Geometry check sheet. Reference: the model listing, model coordinates, mm. A direction names the side the tool comes from. Coordinates: 2 decimals unless noted, no trailing zeros. Loops run counter-clockwise (first coordinate to the right, second up) from the corner with the lowest first, then second, coordinate; pieces in that order, holes last.
from build123d import *

# Parameters (mm, degrees)
SKETCH1_W           = 15
SKETCH1_H           = 15
BOSS_EXTRUDE1_DEPTH = 93
SKETCH2_R           = 3
BOSS_EXTRUDE2_DEPTH = 7
SKETCH3_W           = 3.2
SKETCH3_H           = 2.1
CUT_EXTRUDE1_DEPTH  = 102.396498953
FILLET1_R           = 2
BOSS_EXTRUDE3_START = -5
BOSS_EXTRUDE3_DEPTH = 6
BOSS_EXTRUDE4_DEPTH = 3
BOSS_EXTRUDE5_DEPTH = 9


with BuildPart() as part:
    # Sketch1 → Boss-Extrude1 (new body)
    with BuildSketch(Plane(origin=(0, 0, 0), x_dir=(1, 0, 0), z_dir=(0, 1, 0))):
        Rectangle(SKETCH1_W, SKETCH1_H)
    extrude(amount=BOSS_EXTRUDE1_DEPTH)

    # Sketch2 → Boss-Extrude2 (add)
    with BuildSketch(Plane(origin=(0, 93, 0), x_dir=(1, 0, 0), z_dir=(0, 1, 0))):
        with Locations(Location((1.5, 2.5, 0), (0, 0, 270))):
            Circle(SKETCH2_R)
    extrude(amount=BOSS_EXTRUDE2_DEPTH)

    # Sketch3 → Cut-Extrude1 (cut, through all)
    with BuildSketch(Plane.XY.offset(7.5)):
        with Locations((-5.9, 11.05)):
            Rectangle(SKETCH3_W, SKETCH3_H)
    extrude(amount=-CUT_EXTRUDE1_DEPTH, mode=Mode.SUBTRACT)

    # Fillet1
    fillet1_edges = [part.edges().sort_by_distance(p)[0] for p in [
        (7.5, 46.5, -7.5),
    ]]
    fillet(fillet1_edges, radius=FILLET1_R)

    # Sketch4 → Boss-Extrude3 (add)
    with BuildSketch(Plane.XY.offset(7.5).offset(BOSS_EXTRUDE3_START)):
        Polygon((7.5, 24), (22.5, 24), (22.5, 36), (20.5, 36), (20.5, 27), (7.5, 27), align=None)
    extrude(amount=-BOSS_EXTRUDE3_DEPTH)

    # Sketch5 → Boss-Extrude4 (add)
    with BuildSketch(Plane.XY.offset(2.5)):
        Polygon((20.5, 30), (22.5, 30), (22.5, 24), (7.5, 24), (7.5, 27), (20.5, 27), align=None)
    extrude(amount=BOSS_EXTRUDE4_DEPTH)

    # Sketch6 → Boss-Extrude5 (add)
    with BuildSketch(Plane.XY.offset(5.5)):
        Polygon((22.5, 24), (7.5, 24), (7.5, 9), align=None)
    extrude(amount=-BOSS_EXTRUDE5_DEPTH)


solid = part.part
(1) Scan lines: L1, parallel to X at y = 11.5, z = 2; L2, parallel to Y at x = 0.5, z = 0.75; L3, parallel to Y at x = 19, z = 0.75. Record each from-to range of solid material in increasing order.
Findings:
L1: x = -4.3 to 10
L2: y = 0 to 93
L3: y = 20.5 to 27
(2) Access from +Z, -Z, +X, -X, +Y, -Y to the whole of each face (thin tool, end or side, straight path). Record for faces 1 (the flat face through (21, 30, 4)), 2 (the flat face through (20.5, 31, 0)), 3 (the flat face through (13, 22, 5.5)), 4 (the flat face through (-6, 10, 0)).
Findings:
face 1: +Z, +X, +Y
face 2: +Z, -Z, +Y
face 3: +Z, +X, +Y, -Y
face 4: +Z, -Z, -X
(3) Sectioned sample at D-D on y = 67. Record the cut outline in (x, z), and give its area (3 significant figures).
Findings:
outline: (-7.5, -7.5) - (5.5, -7.5) arc R2 ccw to (7.5, -5.5) - (7.5, 7.5) - (-7.5, 7.5) - close
area: 224 mm2
(4) Sectioned sample at A-A on y = 31. Record the cut outline in (x, z).
Findings:
outline: (-7.5, -7.5) - (5.5, -7.5) arc R2 ccw to (7.5, -5.5) - (7.5, 7.5) - (-7.5, 7.5) - close; (20.5, -3.5) - (22.5, -3.5) - (22.5, 2.5) - (20.5, 2.5) - close
(5) Gauge pin test, flat ends, axial feed: pin 1 Ø3 at (x, z) = (6, -4) entering from +Y; pin 2 Ø0.6 at (y, z) = (11, -3.5) entering from -X; pin 3 Ø8 at (x, z) = (18, 4.5) entering from +Y. Record the tip position at first contact, or that the pin passes through.
Findings:
pin 1: stops at y = 93
pin 2: stops at x = -4.3
pin 3: stops at y = 36
(6) Sectioned sample at C-C on x = 1.5. Record the cut outline in (y, z), and give its area (3 significant figures).
Findings:
outline: (0, -7.5) - (93, -7.5) - (93, -5.5) - (100, -5.5) - (100, 0.5) - (93, 0.5) - (93, 7.5) - (0, 7.5) - close
area: 1,440 mm2
(7) Draft check along X on faces 5 (the flat face through (14, 27, 1)), 6 (the flat face through (22.5, 30, 0)), 7 (the flat face through (-4.3, 11, 0)). Enter one of: +X half, -X half, draft (parallel to the pull), parting line (faces both ways), or undercut.
Findings:
face 5: undercut
face 6: +X half
face 7: -X half
(8) Sectioned sample at B-B on z = -2.5. Record the cut outline in (x, y), and give its area (3 significant figures).
Findings:
outline: (-7.5, 0) - (7.5, 0) - (7.5, 9) - (22.5, 24) - (22.5, 36) - (20.5, 36) - (20.5, 27) - (7.5, 27) - (7.5, 93) - (4.5, 93) - (4.5, 100) - (-1.5, 100) - (-1.5, 93) - (-7.5, 93) - (-7.5, 12.1) - (-4.3, 12.1) - (-4.3, 10) - (-7.5, 10) - close
area: 1,610 mm2
